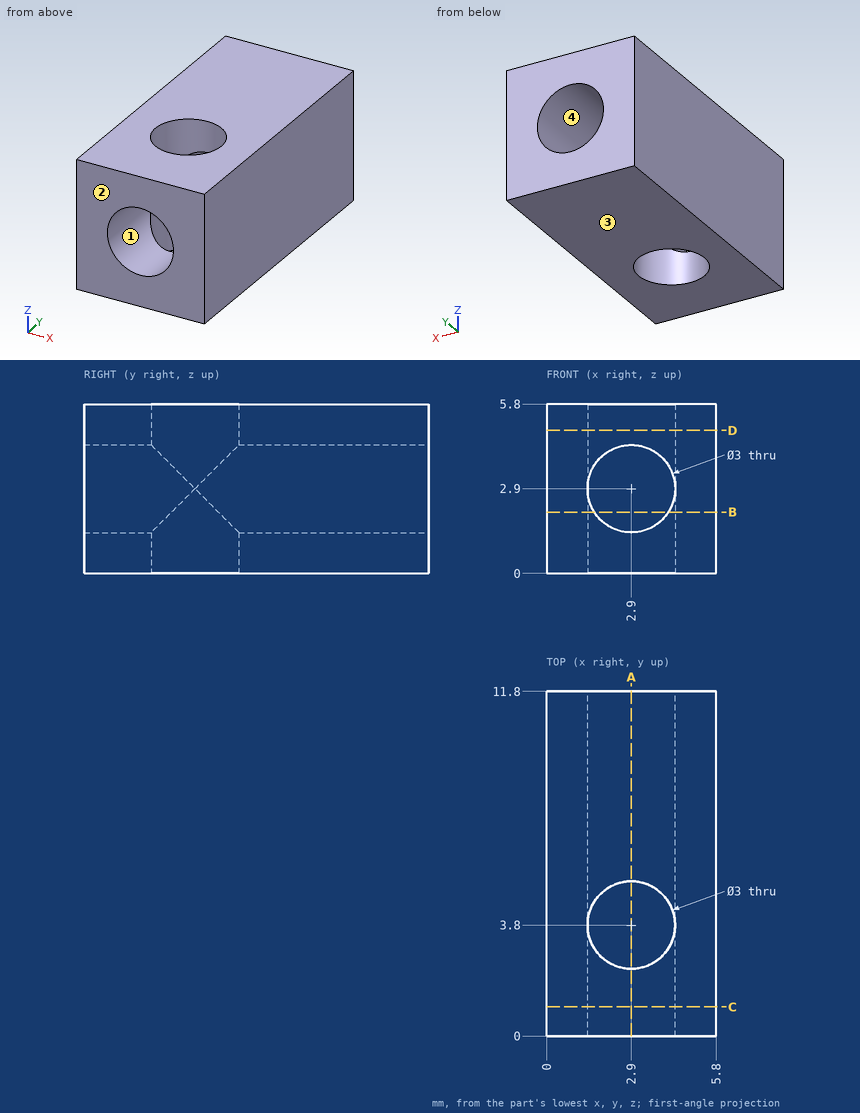
Study the drawing (mm; zero at the part's minimum x, y, z) and answer. Coordinates: 2 decimals unless noted, no trailing zeros. Loops run counter-clockwise (first coordinate to the right, second up) from the corner with the lowest first, then second, coordinate; pieces in that order, holes last. Notation, with made-up numbers: (19, 33) -> (29, 33) arc R28 cw to (29, 68) -> close; hole circle Ø2 at (72.5, 47.25). An arc over 180 degrees is marked (long way). Answer as CSV lines item,"result".
1) The part is cut by section D-D (z = 4.9). Give the vertices of the cut face in (x, y).
A:
outline,"(0, 0) -> (5.8, 0) -> (5.8, 11.8) -> (0, 11.8) -> close; hole circle Ø3 at (2.9, 3.8)"
2) The part is cut by section C-C (y = 1). Give the vertices of the cut face in (x, z), and give its area (3 significant figures).
A:
outline,"(0, 0) -> (5.8, 0) -> (5.8, 5.8) -> (0, 5.8) -> close; hole circle Ø3 at (2.9, 2.9)"
area,"26.6 mm²"
3) The part is cut by section B-B (z = 2.1). Give the vertices of the cut face in (x, y).
A:
outline,"(0, 0) -> (1.63, 0) -> (1.63, 3) arc R1.5 cw to (1.63, 4.6) -> (1.63, 11.8) -> (0, 11.8) -> close; (4.17, 0) -> (5.8, 0) -> (5.8, 11.8) -> (4.17, 11.8) -> (4.17, 4.6) arc R1.5 cw to (4.17, 3) -> close"
4) Straight lines are drawn through the part: probe 1 along X at (y, z) = (5.5, 2.8); probe 2 along Y at (x, z) = (2.8, 1). For each, find the intervals that lie inside material, in ascending order.
A:
probe 1,"x = 0 to 1.4, 4.4 to 5.8"
probe 2,"y = 0 to 2.3, 5.3 to 11.8"
5) For a pull along Z with two mould halves and no side action, classify the marked faces 1, 2, 3 and 4 as released by +Z, released by -Z, zero draft, split by the parting line, or undercut.
A:
face 1,"undercut"
face 2,"zero draft"
face 3,"released by -Z"
face 4,"undercut"
6) The part is cut by section A-A (x = 2.9). Give the vertices of the cut face in (y, z).
A:
outline,"(0, 0) -> (2.3, 0) -> (2.3, 1.4) -> (0, 1.4) -> close; (0, 4.4) -> (2.3, 4.4) -> (2.3, 5.8) -> (0, 5.8) -> close; (5.3, 0) -> (11.8, 0) -> (11.8, 1.4) -> (5.3, 1.4) -> close; (5.3, 4.4) -> (11.8, 4.4) -> (11.8, 5.8) -> (5.3, 5.8) -> close"
